from build123d import *

# Parameters (mm, degrees)
SKETCH1_W           = 350
SKETCH1_H           = 500
SKETCH1_R           = 3
SKETCH1_R_2         = 2.5
SKETCH1_R_3         = 12.665
SKETCH1_W_2         = 200
SKETCH1_H_2         = 49.2
BOSS_EXTRUDE1_DEPTH = 5


with BuildPart() as part:
    # Sketch1 → Boss-Extrude1 (new body)
    with BuildSketch(Plane.XY):
        Rectangle(SKETCH1_W, SKETCH1_H)
        with Locations((-165, 0)):
            Circle(SKETCH1_R, mode=Mode.SUBTRACT)
        with Locations((165, -240)):
            Circle(SKETCH1_R, mode=Mode.SUBTRACT)
        with Locations((165, 0)):
            Circle(SKETCH1_R, mode=Mode.SUBTRACT)
        with Locations((165, 240)):
            Circle(SKETCH1_R, mode=Mode.SUBTRACT)
        with Locations((0, 240)):
            Circle(SKETCH1_R, mode=Mode.SUBTRACT)
        with Locations((0, -240)):
            Circle(SKETCH1_R, mode=Mode.SUBTRACT)
        with Locations((-165, 240)):
            Circle(SKETCH1_R, mode=Mode.SUBTRACT)
        with Locations((-165, -240)):
            Circle(SKETCH1_R, mode=Mode.SUBTRACT)
        with Locations((40, 205)):
            Circle(SKETCH1_R, mode=Mode.SUBTRACT)
        with Locations((0, 205)):
            Circle(SKETCH1_R, mode=Mode.SUBTRACT)
        with Locations((-40, 205)):
            Circle(SKETCH1_R, mode=Mode.SUBTRACT)
        with Locations((0, 130.4)):
            Circle(SKETCH1_R_2, mode=Mode.SUBTRACT)
        with Locations((40, 130.4)):
            Circle(SKETCH1_R_2, mode=Mode.SUBTRACT)
        with Locations((-40, 130.4)):
            Circle(SKETCH1_R_2, mode=Mode.SUBTRACT)
        with Locations((115, -90)):
            Circle(SKETCH1_R_2, mode=Mode.SUBTRACT)
        with Locations((85, -90)):
            Circle(SKETCH1_R_2, mode=Mode.SUBTRACT)
        with Locations((115, -160)):
            Circle(SKETCH1_R_2, mode=Mode.SUBTRACT)
        with Locations((85, -160)):
            Circle(SKETCH1_R_2, mode=Mode.SUBTRACT)
        with Locations((100, -105)):
            Circle(SKETCH1_R_3, mode=Mode.SUBTRACT)
        with Locations((0, 165.4)):
            Rectangle(SKETCH1_W_2, SKETCH1_H_2, mode=Mode.SUBTRACT)
    extrude(amount=BOSS_EXTRUDE1_DEPTH)


solid = part.part
Design review of the part built by this model. Coordinates are the model's own, in mm. Give positions to 0.01 mm unless a question says otherwise; leave off trailing zeros. Write each loop counter-clockwise with the first axis right and the second up, starting at its lowest first coordinate (ties: lowest second). Pieces come first, ordered by that corner, then holes. Notation, with made-up numbers: M -32.75,47.5 L 21.25,47.5 A24 cw 21.25,80.5 Z; hole C 83,-37.75 d5. An arc over 180 degrees is marked long. Return JSON: item names as keys, results as strings. Group by question number.
Item 1: Wall thickness on line 1 along X through (y, z) = (130.4, 1.7); line 2 along Y through (x, z) = (115, 2.3); line 3 along X through (y, z) = (-240, 1): over which ranges is each line inside the solid? List them lowest first.
Item 2: Clearance check with flat-ended pins moving along their axes: pin 1 Ø1.5 at (x, y) = (132.5, -63.5) entering from -Z; pin 2 Ø5.5 at (x, y) = (0, -240) entering from +Z. State where each tip first meets the part, or that it passes through.
Item 3: Take a section at A-A (x = 56.5). Give the boundary of the cut face in (y, z).
Item 4: Take a section at B-B (z = 1.8). Count the separate pieces of the cut face and the enclosed holes in it, plus the area to 3 significant figures.
Item 5: The part is to be moulded in two halves that separate along X. For faces 1 (the cylindrical face through (112.08, -101.2, 2.46)), 2 (the flat face through (-2, 4, 5)), say which applies: pulls with the +X half, pulls with the -X half, needs draft (parallel to the pull), parting line crosses it, or undercut.
Return value:
{
 "1": {"line 1": "x = -175 to -42.5, -37.5 to -2.5, 2.5 to 37.5, 42.5 to 175", "line 2": "y = -250 to -162.5, -157.5 to -92.5, -87.5 to 250", "line 3": "x = -175 to -168, -162 to -3, 3 to 162, 168 to 175"},
 "2": {"pin 1": "stops at z = 0", "pin 2": "passes through"},
 "3": {"outline": "M -250,0 L 140.8,0 L 140.8,5 L -250,5 Z; M 190,0 L 250,0 L 250,5 L 190,5 Z"},
 "4": {"separate pieces": "1", "enclosed holes": "20", "area": "164,000 mm2"},
 "5": {"face 1": "undercut", "face 2": "needs draft"}
}
